Geometry: final body of the model. Coordinates: model frame, mm. A direction names the side the tool comes from. Round coordinates to 2 decimals unless told otherwise and drop trailing zeros. Loops run counter-clockwise (first coordinate to the right, second up) from the corner with the lowest first, then second, coordinate; pieces in that order, holes last. Notation, with made-up numbers: (7.25, 43.5) -> (57.25, 43.5) arc R4 ccw to (57.25, 48.5) -> close; hole circle Ø7 at (-30.5, 52.25). An arc over 180 degrees is marked (long way). Answer in a Markdown table with one row per item.
```python
from build123d import *

# Parameters (mm, degrees)
EXTRUDE_1_DEPTH     = 10
EXTRUDE_2_DEPTH     = 2
CUT_EXTRUDE_1_DEPTH = 5
SKETCH_4_W          = 2.5
SKETCH_4_H          = 6
EXTRUDE_3_DEPTH     = 2.5


with BuildPart() as part:
    # Эскиз1 → Бобышка-Вытянуть1 (new body, symmetric)
    with BuildSketch(Plane.XY):
        Polygon((0, 28), (0, 0), (28, 0), (28, 4), (4, 4), (4, 28), align=None)
    extrude(amount=EXTRUDE_1_DEPTH, both=True)

    # Эскиз2 → Бобышка-Вытянуть2 (add)
    with BuildSketch(Plane.XY.offset(10)):
        Polygon((4, 28), (28, 4), (4, 4), align=None)
    extrude_2 = extrude(amount=-EXTRUDE_2_DEPTH)

    # Зеркальное отражение2: Бобышка-Вытянуть2 across plane
    add(extrude_2.mirror(Plane.XY))

    # Эскиз3 → Вырез-Вытянуть1 (cut, through all)
    with BuildSketch(Plane(origin=(0, 4, 0), x_dir=(1, 0, 0), z_dir=(0, 1, 0))):
        with BuildLine():
            Line((12, 2.5), (18, 2.5))
            ThreePointArc((18, 2.5), (20.5, 0), (18, -2.5))
            Line((18, -2.5), (12, -2.5))
            ThreePointArc((12, -2.5), (9.5, 0), (12, 2.5))
        make_face()
    cut_extrude_1 = extrude(amount=-CUT_EXTRUDE_1_DEPTH, mode=Mode.SUBTRACT)

    # Эскиз4 → Бобышка-Вытянуть3 (add)
    with BuildSketch(Plane.XZ):
        with Locations((4.25, 0)):
            Rectangle(SKETCH_4_W, SKETCH_4_H)
        with Locations((23.75, 0)):
            Rectangle(SKETCH_4_W, SKETCH_4_H)
    extrude_3 = extrude(amount=EXTRUDE_3_DEPTH)

    # Зеркальное отражение3: Вырез-Вытянуть1, Бобышка-Вытянуть3 across plane
    add(cut_extrude_1.mirror(Plane(origin=(0, 0, 0), x_dir=(0, 0, 1), z_dir=(-0.707106781, 0.707106781, 0))), mode=Mode.SUBTRACT)
    add(extrude_3.mirror(Plane(origin=(0, 0, 0), x_dir=(0, 0, 1), z_dir=(-0.707106781, 0.707106781, 0))))


solid = part.part
```
Item 1: Cut plane D-D (x = 0.5). Output: boundary loops of the cut face in (y, z), then the cut area to 3 significant figures.
Answer:
| item | result |
|---|---|
| outline | (0, -10) -> (28, -10) -> (28, 10) -> (0, 10) -> close; hole (12, -2.5) -> (18, -2.5) arc R2.5 ccw to (18, 2.5) -> (12, 2.5) arc R2.5 ccw to start |
| area | 510 mm² |
Item 2: Cut plane C-C (x = 26.5). Output: boundary loops of the cut face in (y, z), then the cut area to 3 significant figures.
Answer:
| item | result |
|---|---|
| outline | (0, -10) -> (5.5, -10) -> (5.5, -8) -> (4, -8) -> (4, 8) -> (5.5, 8) -> (5.5, 10) -> (0, 10) -> close |
| area | 86.0 mm² |
Item 3: Line query: probe 1 along Z at (x, y) = (13, 0.5); probe 2 along Y at (x, z) = (-1, 2.25); probe 3 along Y at (x, z) = (3.5, -8). Output: solid intervals per line, ascending. Write a range as [from, to].
Answer:
| item | result |
|---|---|
| probe 1 | z = [-10, -2.5], [2.5, 10] |
| probe 2 | y = [3, 5.5], [22.5, 25] |
| probe 3 | y = [0, 28] |
Item 4: Cut plane A-A (z = 0). Count the separate pieces of the cut face and the enclosed holes in it, then the cut area to 3 significant figures.
Answer:
| item | result |
|---|---|
| separate pieces | 3 |
| enclosed holes | 0 |
| area | 145 mm² |
Item 5: Draft query along Y for faces 4 (the face through (11, 11, -10)), 5 (the face through (-1, 5.5, 0)), 6 (the face through (4, -2.5, 0)). Return one class per face: pulls with the +Y half, pulls with the -Y half, needs draft (parallel to the pull), parting line crosses it, or undercut.
Answer:
| item | result |
|---|---|
| face 4 | needs draft |
| face 5 | undercut |
| face 6 | pulls with the -Y half |
Item 6: Reachability of faces 1 (the face through (-1, 4, 3)), 2 (the face through (15, 2, 2.5)), 3 (the face through (24, -1, -3)) from +Z, -Z, +X, -X, +Y, -Y: full face, straight path, thin tool, end or side. Return the list, or none.
Answer:
| item | result |
|---|---|
| face 1 | +Z, -X, +Y, -Y |
| face 2 | +Y, -Y |
| face 3 | -Z, +X, -X, -Y |
Item 7: Pin query (flat end, axial travel): pin 1 Ø1 at (y, z) = (24, 7) entering from +X; pin 2 Ø1.3 at (x, y) = (-1.5, 23.5) entering from -Z; pin 3 Ø1.2 at (x, y) = (23.5, -1) entering from +Z. Return the tip coordinate at first contact, or that it passes through.
Answer:
| item | result |
|---|---|
| pin 1 | stops at x = 4 |
| pin 2 | stops at z = -3 |
| pin 3 | stops at z = 3 |
Item 8: Cut plane B-B (y = 20). Output: boundary loops of the cut face in (x, z).
Answer:
| item | result |
|---|---|
| outline | (0, -10) -> (12, -10) -> (12, -8) -> (4, -8) -> (4, -1.5) -> (0, -1.5) -> close; (0, 1.5) -> (4, 1.5) -> (4, 8) -> (12, 8) -> (12, 10) -> (0, 10) -> close |
